from build123d import *

# Parameters (mm, degrees)
BOSS_EXTRUDE1_DEPTH          = 3.175
CUT_EXTRUDE1_START           = -3.175
CUT_EXTRUDE1_DEPTH           = 3.175
F_2_5_2_5_DIAMETER_HOLE1_D   = 2.5
F_22_0_22_DIAMETER_HOLE1_D   = 22
F_10_5_10_5_DIAMETER_HOLE1_D = 10.5
F_5_2_5_2_DIAMETER_HOLE1_D   = 5.2


with BuildPart() as part:
    # Sketch1 → Boss-Extrude1 (new body)
    with BuildSketch(Plane(origin=(0, 73.175, 0), x_dir=(1, 0, 0), z_dir=(0, 1, 0))):
        with BuildLine():
            Line((15, -131.043137062), (-1.022023545, -131.043137062))
            ThreePointArc((-1.022023545, -131.043137062), (-0.325892642, -137.979342107), (-4.330946321, -143.685048347))
            ThreePointArc((-4.330946321, -143.685048347), (-7.347711019, -143.543683532), (-9.490358424, -145.672043312))
            ThreePointArc((-9.490358424, -145.672043312), (-16, -155.043137062), (-9.490358424, -164.414230812))
            ThreePointArc((-9.490358424, -164.414230812), (-7.347711019, -166.542590592), (-4.330946321, -166.401225777))
            ThreePointArc((-4.330946321, -166.401225777), (-1.426295687, -166.532567239), (0, -169.066324625))
            Line((0, -169.066324625), (0, -171.243137062))
            ThreePointArc((0, -171.243137062), (1.40588745, -174.637249612), (4.8, -176.043137062))
            Line((4.8, -176.043137062), (15.2, -176.043137062))
            ThreePointArc((15.2, -176.043137062), (18.59411255, -174.637249612), (20, -171.243137062))
            Line((20, -171.243137062), (20, -170.064478312))
            ThreePointArc((20, -170.064478312), (21.68082981, -167.69523564), (24.452536205, -168.564800671))
            ThreePointArc((24.452536205, -168.564800671), (28.846907451, -169.817736591), (31.189498771, -165.894394524))
            ThreePointArc((31.189498771, -165.894394524), (31.338525975, -164.871140606), (31.978698654, -164.05908357))
            ThreePointArc((31.978698654, -164.05908357), (37.999904187, -151.989523925), (31.892574785, -139.963314477))
            ThreePointArc((31.892574785, -139.963314477), (31.188720102, -139.008164704), (31.149849359, -137.822326786))
            ThreePointArc((31.149849359, -137.822326786), (28.808294112, -133.301045501), (24.117695109, -135.281738919))
            ThreePointArc((24.117695109, -135.281738919), (22.762301061, -136.401892346), (21.046177665, -136.018803304))
            ThreePointArc((21.046177665, -136.018803304), (20.21083435, -135.158715929), (19.614707675, -134.118436286))
            ThreePointArc((19.614707675, -134.118436286), (17.772769024, -131.882397712), (15, -131.043137062))
        make_face()
    extrude(amount=-BOSS_EXTRUDE1_DEPTH)

    # Sketch2 → Cut-Extrude1 (cut)
    with BuildSketch(Plane.XZ.offset(-70).offset(CUT_EXTRUDE1_START)):
        with BuildLine():
            Line((0, 136.043137062), (0, 135.44721912))
            ThreePointArc((0, 135.44721912), (-0.258856213, 133.18666217), (-1.022023545, 131.043137062))
            Line((-1.022023545, 131.043137062), (5, 131.043137062))
            ThreePointArc((5, 131.043137062), (1.464466094, 132.507603156), (0, 136.043137062))
        make_face()
    extrude(amount=CUT_EXTRUDE1_DEPTH, mode=Mode.SUBTRACT)

    # Ø2.5 (2.5) Diameter Hole1 (through all)
    with Locations(Plane(origin=(0, 73.175, 0), x_dir=(1, 0, 0), z_dir=(0, 1, 0))):
        with Locations((27.534095489, -136.827930511), (27.465074328, -166.331615936), (-6, -147.043137062), (-6, -163.043137062)):
            Hole(F_2_5_2_5_DIAMETER_HOLE1_D / 2)

    # Ø22.0 (22) Diameter Hole1 (through all)
    with Locations(Plane(origin=(0, 73.175, 0), x_dir=(1, 0, 0), z_dir=(0, 1, 0))):
        with Locations((23, -152.043137062)):
            Hole(F_22_0_22_DIAMETER_HOLE1_D / 2)

    # Ø10.5 (10.5) Diameter Hole1 (through all)
    with Locations(Plane(origin=(0, 73.175, 0), x_dir=(1, 0, 0), z_dir=(0, 1, 0))):
        with Locations((-6, -155.043137062)):
            Hole(F_10_5_10_5_DIAMETER_HOLE1_D / 2)

    # Ø5.2 (5.2) Diameter Hole1 (through all)
    with Locations(Plane(origin=(0, 73.175, 0), x_dir=(1, 0, 0), z_dir=(0, 1, 0))):
        with Locations((10, -171.043137062), (10, -136.043137062)):
            Hole(F_5_2_5_2_DIAMETER_HOLE1_D / 2)


solid = part.part
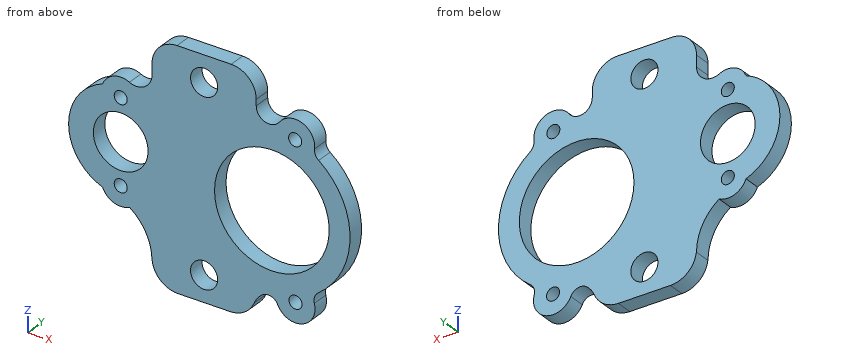
CAD build for the part. Positions are in the model's coordinates, mm. Give positions to 0.01 mm unless a question says otherwise; leave off trailing zeros. Order: outer loops, then holes, each group sorted by start corner. A loop starts at its lowest first (then second) coordinate and runs counter-clockwise, first axis right, second up. Notation, with made-up numbers: (17, 22.25) - (48, 22.25) arc R30 ccw to (48, 49.25) - close; hole circle Ø2 at (-38.5, 67.25). An arc over 180 degrees is marked (long way). Answer in a Markdown table with one row per item.
1. Saw through at D-D, the plane y = 70.9. Count the separate pieces of the cut face and the enclosed holes in it, plus the area to 3 significant figures.
Data:
| item | result |
|---|---|
| separate pieces | 1 |
| enclosed holes | 8 |
| area | 1,170 mm² |
2. Saw through at C-C, the plane z = 173. Give the cut face in (x, y) (3 decimals).
Data:
| item | result |
|---|---|
| outline | (0.333, 70) - (8.288, 70) - (8.288, 73.175) - (0.333, 73.175) - close; (11.712, 70) - (19.667, 70) - (19.667, 73.175) - (11.712, 73.175) - close |
3. Saw through at B-B, the plane x = -6. Give the cut face in (y, z) (3 decimals).
Data:
| item | result |
|---|---|
| outline | (70, 143.293) - (73.175, 143.293) - (73.175, 145.793) - (70, 145.793) - close; (70, 148.293) - (73.175, 148.293) - (73.175, 149.793) - (70, 149.793) - close; (70, 160.293) - (73.175, 160.293) - (73.175, 161.793) - (70, 161.793) - close; (70, 164.293) - (73.175, 164.293) - (73.175, 166.793) - (70, 166.793) - close |
4. Probe probe 1 along Z at (x, y) = (-6, 72.3); probe 2 along Z at (x, y) = (10, 71.2); probe 3 along X at (y, z) = (71.4, 147.5). List the from-to ranges inside material, lowest first. Write a range as [from, to].
Data:
| item | result |
|---|---|
| probe 1 | z = [143.29, 145.79], [148.29, 149.79], [160.29, 161.79], [164.29, 166.79] |
| probe 2 | z = [131.04, 133.44], [138.64, 168.44], [173.64, 176.04] |
| probe 3 | x = [-12.57, -7.16], [-4.84, 12.98], [33.02, 37.3] |
5. Saw through at A-A, the plane x = 10. Give the cut face in (y, z) (3 decimals).
Data:
| item | result |
|---|---|
| outline | (70, 131.043) - (73.175, 131.043) - (73.175, 133.443) - (70, 133.443) - close; (70, 138.643) - (73.175, 138.643) - (73.175, 168.443) - (70, 168.443) - close; (70, 173.643) - (73.175, 173.643) - (73.175, 176.043) - (70, 176.043) - close |
6. Flat gauge pins, fed straight in: pin 1 (1 mm diameter, centred on y = 72.5, z = 153.5, fed in from +X); pin 2 (0.7 mm diameter, centred on y = 71.5, z = 170, fed in from -X). Where does each tip first touch, or does it go through?
Data:
| item | result |
|---|---|
| pin 1 | stops at x = 37.97 |
| pin 2 | stops at x = 0 |
